The model under review builds one solid part; all positions refer to its coordinate system, in mm. Face numbers are marked on the shaded views. A direction names the side the tool comes from. Give positions to 0.01 mm unless a question says otherwise; leave off trailing zeros. Write each loop counter-clockwise with the first axis right and the second up, starting at its lowest first coordinate (ties: lowest second). Pieces come first, ordered by that corner, then holes. Notation, with made-up numbers: (67, 34.25) - (89, 34.25) arc R11 cw to (89, 51.25) - close; hole circle Ø2 at (-2.75, -10). An arc over 180 degrees is marked (long way). Write item = value, one per line.
```python
from build123d import *

# Parameters (mm, degrees)
F0_W     = 99.06
F0_H     = 99.06
F1_DEPTH = 25.4
F2_T     = -0.889
F3_W     = 81.28
F3_H     = 81.28
F4_DEPTH = 16.51
F5_W     = 79.502
F5_H     = 79.502
F6_DEPTH = 16.51


with BuildPart() as f1:
    # F0 (on Top) → F1 (new body)
    with BuildSketch(Plane.XY):
        Rectangle(F0_W, F0_H)
    extrude(amount=F1_DEPTH)

    # F2
    f2_openings = [f1.faces().sort_by_distance(p)[0] for p in [
        (0, 0, 25.4),
    ]]
    offset(amount=F2_T, openings=f2_openings)

    # F3 (on face) → F4 (join)
    with BuildSketch(Plane.XY.offset(0.889)):
        Rectangle(F3_W, F3_H)
    extrude(amount=F4_DEPTH)

    # F5 (on face) → F6 (cut)
    with BuildSketch(Plane(origin=(0, 0, 0), x_dir=(1, 0, 0), z_dir=(0, 0, -1))):
        Rectangle(F5_W, F5_H)
    extrude(amount=-F6_DEPTH, mode=Mode.SUBTRACT)


solid = f1.part
```
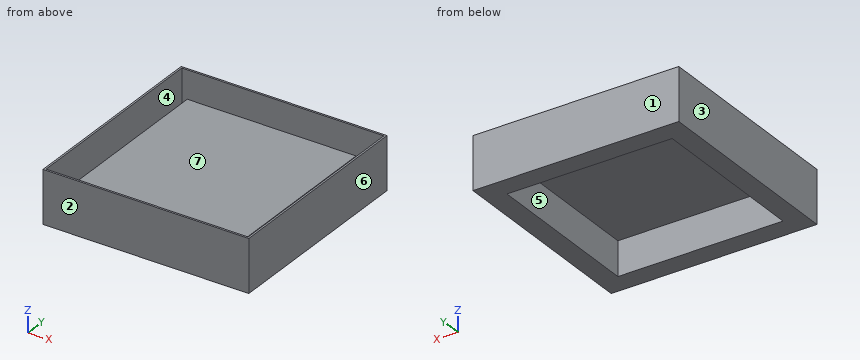
1. Take a section at B-B on z = 22.5. Give the boundary of the cut face in (x, y), and give its area (3 significant figures).
Findings below:
outline = (-49.53, -49.53) - (49.53, -49.53) - (49.53, 49.53) - (-49.53, 49.53) - close; hole (-48.64, -48.64) - (48.64, -48.64) - (48.64, 48.64) - (-48.64, 48.64) - close
area = 349 mm²
2. Insertion check: P1, Ø12, axis at x = -7, y = -12, coming from the +Z side; P2, Ø1, axis at x = -33, y = -27, coming from the -Z side. Each pin has a flat end and moves straight along its axis. Give the tip position at first contact, or say it passes through.
Findings below:
P1 = 17.4
P2 = 16.51
3. Take a section at A-A on z = 14.25. Give the boundary of the cut face in (x, y).
Findings below:
outline = (-49.53, -49.53) - (49.53, -49.53) - (49.53, 49.53) - (-49.53, 49.53) - close; (-40.64, -40.64) - (40.64, -40.64) - (40.64, 40.64) - (-40.64, 40.64) - close; hole (-48.64, -48.64) - (48.64, -48.64) - (48.64, 48.64) - (-48.64, 48.64) - close; hole (-39.75, -39.75) - (39.75, -39.75) - (39.75, 39.75) - (-39.75, 39.75) - close
4. Draft analysis for pull direction Y (two halves, no side actions). For the marked faces 1, 2, 3 and 4, state which applies: +Y half, -Y half, draft (parallel to the pull), parting line (faces both ways), or undercut.
Findings below:
face_1 = +Y half
face_2 = -Y half
face_3 = draft
face_4 = undercut
5. Take a section at C-C on y = -13. Give the boundary of the cut face in (x, z), and give its area (3 significant figures).
Findings below:
outline = (-49.53, 0) - (-39.75, 0) - (-39.75, 16.51) - (39.75, 16.51) - (39.75, 0) - (49.53, 0) - (49.53, 25.4) - (48.64, 25.4) - (48.64, 0.89) - (40.64, 0.89) - (40.64, 17.4) - (-40.64, 17.4) - (-40.64, 0.89) - (-48.64, 0.89) - (-48.64, 25.4) - (-49.53, 25.4) - close
area = 161 mm²
6. For line 1 (X direction, y = 27, z = 15.5); line 2 (X direction, y = 40, z = 13.75), list the stretches that pass through material, from the lowest coordinate up. Write a range as from..to.
Findings below:
line_1 = -49.53..-48.64, -40.64..-39.75, 39.75..40.64, 48.64..49.53
line_2 = -49.53..-48.64, -40.64..40.64, 48.64..49.53
7. Machinability: for the marked faces 5, 6 and 7, which of the approach directions +Z, -Z, +X, -X, +Y, -Y give a long, thin tool a straight path to every point of the face, cutting with its end or side? Answer none if there is none.
Findings below:
face_5 = -Z
face_6 = +Z, -Z, +X, +Y, -Y
face_7 = +Z
